The listing builds one solid part. Answer for the finished solid, in the listing's coordinates (mm). A direction names the side the tool comes from. Coordinates: 2 decimals unless noted, no trailing zeros. Write each loop counter-clockwise with the first axis right and the second up, starting at its lowest first coordinate (ties: lowest second). Pieces come first, ordered by that corner, then holes.
from build123d import *

# Parameters (mm, degrees)
BASE_FLANGE1_DEPTH      = 406.4
CUT_EXTRUDE1_START      = -88.9254
CUT_EXTRUDE1_OUTLINE_W  = 324.85
CUT_EXTRUDE1_OUTLINE_H  = 158.75
CUT_EXTRUDE1_DEPTH      = 88.9254
CUT_EXTRUDE2_REACH      = 763.365
CUT_EXTRUDE3_REACH      = 763.365
SKETCH5_W               = 76.2
SKETCH5_H               = 88.9
CUT_EXTRUDE4_REACH      = 778.597
SKETCH6_W               = 25.4
SKETCH6_H               = 50.8
CUT_EXTRUDE5_REACH      = 793.41
SKETCH8_W               = 31.8008
SKETCH8_H               = 50.8
SKETCH9_W               = 203.2
SKETCH9_H               = 50.8
CUT_EXTRUDE6_DEPTH      = 792.409750066
CUT_EXTRUDE8_DEPTH      = 757.396689906
CUT_EXTRUDE8_DEPTH_BACK = 757.396689906


# Read off the part's stored shape, not the designer's step: Cut-Extrude1
# Sheet-metal steps are written as plain solids
with BuildPart() as part:
    # Sketch2 → Base-Flange1 (new body)
    with BuildSketch(Plane(origin=(0, 0, 0), x_dir=(1, 0, 0), z_dir=(0, 1, 0))):
        with BuildLine():
            Line((596.9, 241.3), (596.9, -38.0746))
            ThreePointArc((596.9, -38.0746), (595.032688573, -42.582688573), (590.5246, -44.45))
            Line((590.5246, -44.45), (527.0754, -44.45))
            ThreePointArc((527.0754, -44.45), (527.057439485, -44.457439486), (527.05, -44.4754))
            Line((527.05, -44.4754), (527.05, -76.1746))
            ThreePointArc((527.05, -76.1746), (525.182688573, -80.682688573), (520.6746, -82.55))
            Line((520.6746, -82.55), (304.8254, -82.55))
            ThreePointArc((304.8254, -82.55), (300.317311427, -80.682688573), (298.45, -76.1746))
            Line((298.45, -76.1746), (298.45, -0.0254))
            ThreePointArc((298.45, -0.0254), (298.442560512, -0.007439487), (298.4246, 0))
            Line((298.4246, 0), (6.3754, 0))
            ThreePointArc((6.3754, 0), (1.867311427, 1.867311427), (0, 6.3754))
            Line((0, 6.3754), (0, 241.3))
            Line((0, 241.3), (6.35, 241.3))
            Line((6.35, 241.3), (6.35, 6.3754))
            ThreePointArc((6.35, 6.3754), (6.357439488, 6.357439488), (6.3754, 6.35))
            Line((6.3754, 6.35), (298.424685325, 6.35))
            ThreePointArc((298.424685325, 6.35), (302.932718863, 4.482658283), (304.8, -0.025400347))
            Line((304.8, -0.025400347), (304.8, -76.1746))
            ThreePointArc((304.8, -76.1746), (304.807439488, -76.192560512), (304.8254, -76.2))
            Line((304.8254, -76.2), (520.6746, -76.2))
            ThreePointArc((520.6746, -76.2), (520.692560512, -76.192560512), (520.7, -76.1746))
            Line((520.7, -76.1746), (520.7, -44.47559657))
            ThreePointArc((520.7, -44.47559657), (522.567241925, -39.967380926), (527.075399994, -38.1))
            Line((527.075399994, -38.1), (590.5246, -38.1))
            ThreePointArc((590.5246, -38.1), (590.542560512, -38.092560512), (590.55, -38.0746))
            Line((590.55, -38.0746), (590.55, 241.3))
            Line((590.55, 241.3), (596.9, 241.3))
        make_face()
    extrude(amount=BASE_FLANGE1_DEPTH)

    # Cut-Extrude1 outline → Cut-Extrude1 (cut)
    with BuildSketch(Plane.XY.offset(82.55).offset(CUT_EXTRUDE1_START)):
        with Locations((161.425, 79.375)):
            Rectangle(CUT_EXTRUDE1_OUTLINE_W, CUT_EXTRUDE1_OUTLINE_H)
    extrude(amount=CUT_EXTRUDE1_DEPTH, mode=Mode.SUBTRACT)

    # Sketch4 → Cut-Extrude2 (cut, up to next)
    with BuildSketch(Plane.ZY, mode=Mode.PRIVATE) as cut_extrude2_sk1:
        Polygon((-241.3, 0), (-6.3754, 0), (-6.3754, 139.7), (-82.5754, 139.7), (-82.5754, 88.9), (-241.3, 88.9), align=None)
    cut_extrude2_tool1 = extrude(cut_extrude2_sk1.sketch, amount=-CUT_EXTRUDE2_REACH, mode=Mode.PRIVATE) & part.part
    add(cut_extrude2_tool1.solids().sort_by_distance((0, 55.372169, -111.42813))[0], mode=Mode.SUBTRACT)

    # Sketch5 → Cut-Extrude3 (cut, up to next)
    with BuildSketch(Plane(origin=(596.9, 0, 0), x_dir=(0, 0, -1), z_dir=(1, 0, 0)), mode=Mode.PRIVATE) as cut_extrude3_sk1:
        with Locations((203.2, 44.45)):
            Rectangle(SKETCH5_W, SKETCH5_H)
    cut_extrude3_tool1 = extrude(cut_extrude3_sk1.sketch, amount=-CUT_EXTRUDE3_REACH, mode=Mode.PRIVATE) & part.part
    add(cut_extrude3_tool1.solids().sort_by_distance((596.9, 44.45, -203.2))[0], mode=Mode.SUBTRACT)

    # Sketch6 → Cut-Extrude4 (cut, up to next)
    with BuildSketch(Plane.XY.offset(44.45), mode=Mode.PRIVATE) as cut_extrude4_sk1:
        with Locations((539.7754, 25.4)):
            Rectangle(SKETCH6_W, SKETCH6_H)
    cut_extrude4_tool1 = extrude(cut_extrude4_sk1.sketch, amount=-CUT_EXTRUDE4_REACH, mode=Mode.PRIVATE) & part.part
    add(cut_extrude4_tool1.solids().sort_by_distance((539.7754, 25.4, 44.45))[0], mode=Mode.SUBTRACT)

    # Sketch8 → Cut-Extrude5 (cut, up to next)
    with BuildSketch(Plane.XY.offset(82.55), mode=Mode.PRIVATE) as cut_extrude5_sk1:
        with Locations((536.575, 25.4)):
            Rectangle(SKETCH8_W, SKETCH8_H)
    cut_extrude5_tool1 = extrude(cut_extrude5_sk1.sketch, amount=-CUT_EXTRUDE5_REACH, mode=Mode.PRIVATE) & part.part
    add(cut_extrude5_tool1.solids().sort_by_distance((536.575, 25.4, 82.55))[0], mode=Mode.SUBTRACT)

    # Sketch9 → Cut-Extrude6 (cut, through all)
    with BuildSketch(Plane.XY.offset(82.55)):
        with Locations((419.0746, 381)):
            Rectangle(SKETCH9_W, SKETCH9_H)
    extrude(amount=-CUT_EXTRUDE6_DEPTH, mode=Mode.SUBTRACT)

    # Sketch11 → Cut-Extrude8 (cut, two sides: drawn at the far end of the back side and taken through both)
    with BuildSketch(Plane(origin=(6.35, 0, 0), x_dir=(0, 0, -1), z_dir=(1, 0, 0)).offset(-CUT_EXTRUDE8_DEPTH_BACK)):
        with BuildLine():
            Line((12.7, 406.4), (12.7, 355.6))
            ThreePointArc((12.7, 355.6), (20.139487758, 337.639487758), (38.1, 330.2))
            Line((38.1, 330.2), (114.3, 330.2))
            ThreePointArc((114.3, 330.2), (132.260512242, 322.760512242), (139.7, 304.8))
            Line((139.7, 304.8), (139.7, 215.9))
            ThreePointArc((139.7, 215.9), (147.139487758, 197.939487758), (165.1, 190.5))
            Line((165.1, 190.5), (241.3, 190.5))
            Line((241.3, 190.5), (241.3, 406.4))
            Line((241.3, 406.4), (12.7, 406.4))
        make_face()
    extrude(amount=CUT_EXTRUDE8_DEPTH + CUT_EXTRUDE8_DEPTH_BACK, mode=Mode.SUBTRACT)


solid = part.part
1. Section A-A on z = -60 is taken. Give the vertices of the cut face in (x, y), then the cut area to 3 significant figures.
Results found:
outline: (0, 139.7) - (6.35, 139.7) - (6.35, 330.2) - (0, 330.2) - close; (590.55, 0) - (596.9, 0) - (596.9, 330.2) - (590.55, 330.2) - close
area: 3,310 mm2
2. Flat-ended cylindrical pins translate along their axes: P1, Ø5, axis at x = 510, y = 319, coming from the -Z side; P2, Ø5, axis at y = 22.5, z = 80.5, coming from the +X side; P3, Ø3, axis at x = 3.5, y = 381, coming from the -Z side. Find the tip coordinate at first contact, or state that the pin passes through.
Results found:
P1: stops at z = 76.2
P2: stops at x = 520.67
P3: stops at z = -12.7
3. A tool of negligible diameter and unlimited length cuts with its end or side. For faces 1 (the flat face through (304.8, 281, 38)), 2 (the flat face through (559, 200, 44.45)), 3 (the flat face through (596.9, 155, -73)), 4 (the flat face through (154, 281, 0)), 5 (the cylindrical face through (593.68, 322.96, -132.06)), from which of +Z, -Z, +X, -X, +Y, -Y can it reach the whole face along a straight path? Write none if from no direction.
Results found:
face 1: -Z, +Y, -Y
face 2: +Z, +X, +Y, -Y
face 3: +Z, -Z, +X, +Y, -Y
face 4: +Z, -X, +Y, -Y
face 5: -Z, +X, -X, +Y
4. For a pull along X with two mould halves and no side action, classify faces 6 (the flat face through (411, 200, 76.2)), 7 (the flat face through (590.55, 155, -69)), 8 (the flat face through (527.05, 226, 60)), 9 (the cylindrical face through (3.13, 322.96, -132.06)) as pulls with the +X half, pulls with the -X half, needs draft (parallel to the pull), parting line crosses it, or undercut.
Results found:
face 6: undercut
face 7: undercut
face 8: pulls with the +X half
face 9: needs draft
5. Section D-D on z = 30.5 is taken. Give the vertices of the cut face in (x, y), then the cut area to 3 significant figures.
Results found:
outline: (298.45, 158.75) - (304.8, 158.75) - (304.8, 406.4) - (298.45, 406.4) - close; (590.55, 0) - (596.9, 0) - (596.9, 406.4) - (590.55, 406.4) - close
area: 4,150 mm2
6. Find the intervals of material crossed by L1, parallel to Z at x = 437.5, y = 30; L2, parallel to X at y = 95, z = -73; L3, parallel to Z at x = 96, y = 294.5, in increasing order.
Results found:
L1: z = 76.2 to 82.55
L2: x = 590.55 to 596.9
L3: z = -6.35 to 0
